from build123d import *

# Parameters (mm, degrees)
SKETCH1_W           = 11
SKETCH1_H           = 4
BOSS_EXTRUDE1_DEPTH = 1.6
SKETCH3_R           = 0.6
CUT_EXTRUDE1_DEPTH  = 1.6
SKETCH2_W           = 0.5
SKETCH2_H           = 1.6
BOSS_EXTRUDE2_DEPTH = 0.01
BOSS_EXTRUDE3_DEPTH = 0.01
SKETCH5_W           = 11
SKETCH5_H           = 1.6
BOSS_EXTRUDE4_DEPTH = 1.5
SKETCH6_W           = 11
SKETCH6_H           = 1.6
BOSS_EXTRUDE5_DEPTH = 0.9


with BuildPart() as part:
    # Sketch1 → Boss-Extrude1 (new body)
    with BuildSketch(Plane(origin=(0, 0, 0), x_dir=(1, 0, 0), z_dir=(0, 1, 0))):
        Rectangle(SKETCH1_W, SKETCH1_H)
    extrude(amount=BOSS_EXTRUDE1_DEPTH)

    # Sketch3 → Cut-Extrude1 (cut)
    with BuildSketch(Plane(origin=(0, 1.6, 0), x_dir=(1, 0, 0), z_dir=(0, 1, 0))):
        with Locations((4.25, 0)):
            Circle(SKETCH3_R)
        with Locations((-4.25, 0)):
            Circle(SKETCH3_R)
    extrude(amount=-CUT_EXTRUDE1_DEPTH, mode=Mode.SUBTRACT)

    # Sketch2 → Boss-Extrude2 (add)
    with BuildSketch(Plane(origin=(0, 1.6, 0), x_dir=(1, 0, 0), z_dir=(0, 1, 0))):
        with Locations((-3, 0)):
            Rectangle(SKETCH2_W, SKETCH2_H)
        with Locations((3, 0)):
            Rectangle(SKETCH2_W, SKETCH2_H)
    extrude(amount=BOSS_EXTRUDE2_DEPTH)

    # Sketch4 → Boss-Extrude3 (add)
    with BuildSketch(Plane(origin=(0, 1.6, 0), x_dir=(1, 0, 0), z_dir=(0, 1, 0))):
        with BuildLine():
            Line((3.25, -0.125), (3.663165, -0.125))
            ThreePointArc((3.663165, -0.125), (3.65, 0), (3.663165, 0.125))
            Line((3.663165, 0.125), (3.25, 0.125))
            Line((3.25, 0.125), (3.25, -0.125))
        make_face()
        with BuildLine():
            Line((-3.25, 0.125), (-3.663165, 0.125))
            ThreePointArc((-3.663165, 0.125), (-3.6533, 0.062846), (-3.65, 0))
            ThreePointArc((-3.65, 0), (-3.6533, -0.062846), (-3.663165, -0.125))
            Line((-3.663165, -0.125), (-3.25, -0.125))
            Line((-3.25, -0.125), (-3.25, 0.125))
        make_face()
    extrude(amount=BOSS_EXTRUDE3_DEPTH)

    # Sketch5 → Boss-Extrude4 (add)
    with BuildSketch(Plane.XY.offset(2)):
        with Locations((0, 0.8)):
            Rectangle(SKETCH5_W, SKETCH5_H)
    extrude(amount=BOSS_EXTRUDE4_DEPTH)

    # Sketch6 → Boss-Extrude5 (add)
    with BuildSketch(Plane(origin=(0, 0, -2), x_dir=(-1, 0, 0), z_dir=(0, 0, -1))):
        with Locations((0, 0.8)):
            Rectangle(SKETCH6_W, SKETCH6_H)
    extrude(amount=BOSS_EXTRUDE5_DEPTH)


solid = part.part
Here's how the part is built. I have some questions about the finished solid (model axes, mm). Coordinates: 2 decimals unless noted, no trailing zeros. Write each loop counter-clockwise with the first axis right and the second up, starting at its lowest first coordinate (ties: lowest second). Pieces come first, ordered by that corner, then holes.
Item 1: If I drill on line 1 (X direction, y = 0.85, z = 0); line 2 (Z direction, x = -4.25, y = 1.1); line 3 (Y direction, x = 2, z = 2), over which ranges is the centre line in solid material (lowest first)?
Item 2: I want a section at A-A on x = 4.25. Write out the boundary of the cut face in (y, z).
Item 3: I want a section at B-B on z = 0.25. Count the separate pieces of the cut face and the enclosed holes in it, and give its area (3 significant figures).
Item 4: I want a section at C-C on y = 0.7. Write out the boundary of the cut face in (x, z), and give its area (3 significant figures).
Item 5: Will these pins go through, and if not, where does the flat tip stop? pin 1 (1.9 mm diameter, centred on x = -4.25, z = 0, fed in from -Y); pin 2 (3 mm diameter, centred on x = -1, z = -0.5, fed in from +Y).
Item 6: If we mould it in two halves opening along Z, with no side actions, what happens to faces 1 (the cylindrical face through (-4.85, 0.81, -0.03)), 2 (the flat face through (0, 1, -2.9)), 3 (the flat face through (-3, 1.61, 0))? For each: +Z half, -Z half, draft (parallel to the pull), parting line (faces both ways), or undercut.
Findings below:
1. line 1: x = -5.5 to -4.85, -3.65 to 3.65, 4.85 to 5.5
1. line 2: z = -2.9 to -0.6, 0.6 to 3.5
1. line 3: y = 0 to 1.6
2. outline: (0, -2.9) - (1.6, -2.9) - (1.6, -0.6) - (0, -0.6) - close; (0, 0.6) - (1.6, 0.6) - (1.6, 3.5) - (0, 3.5) - close
3. separate pieces: 3
3. enclosed holes: 0
3. area: 14.1 mm2
4. outline: (-5.5, -2.9) - (5.5, -2.9) - (5.5, 3.5) - (-5.5, 3.5) - close; hole circle Ø1.2 at (-4.25, 0); hole circle Ø1.2 at (4.25, 0)
4. area: 68.1 mm2
5. pin 1: stops at y = 0
5. pin 2: stops at y = 1.6
6. face 1: undercut
6. face 2: -Z half
6. face 3: draft
